Geometry: final body of the model. Coordinates: model frame, mm. A direction names the side the tool comes from. Round coordinates to 2 decimals unless told otherwise and drop trailing zeros. Write each loop counter-clockwise with the first axis right and the second up, starting at its lowest first coordinate (ties: lowest second). Pieces come first, ordered by that corner, then holes. Notation, with made-up numbers: M 10.5,35 L 66.5,35 A20 cw 66.5,57 Z; hole C 66,80.25 d9. An arc over 180 degrees is marked long. Put each result on its own line as item: value. Start each with the question number.
```python
from build123d import *

# Parameters (mm, degrees)
SKETCH_3_R          = 5
CUT_EXTRUDE_1_DEPTH = 93.736184955
CUT_EXTRUDE_2_DEPTH = 15
CUT_EXTRUDE_3_DEPTH = 15
CUT_EXTRUDE_START   = -15
CUT_EXTRUDE_4_DEPTH = 15
CUT_EXTRUDE_5_DEPTH = 15


with BuildPart() as part:
    # 扫描1: sweep along a path in 草图2
    with BuildLine(Plane.XY) as sweep_1_path:
        CenterArc((0, 0), 50, 0, 360)
    # 草图1 → 扫描1 (sweep)
    with BuildSketch(Plane(origin=(0, 0, 0), x_dir=(1, 0, 0), z_dir=(0, 1, 0))):
        with BuildLine():
            Line((0, 0), (7.5, 0))
            Line((7.5, 0), (7.5, 35))
            ThreePointArc((7.5, 35), (13.357864376, 49.142135624), (27.5, 55))
            Line((27.5, 55), (50, 55))
            Line((50, 55), (50, 60))
            Line((50, 60), (0, 60))
            Line((0, 60), (0, 0))
        make_face()
    sweep(path=sweep_1_path.line)

    # 草图3 → 切除-拉伸1 (cut, through all)
    with BuildSketch(Plane.XY):
        Circle(SKETCH_3_R)
    extrude(amount=-CUT_EXTRUDE_1_DEPTH, mode=Mode.SUBTRACT)

    # 草图5 → 切除-拉伸2 (cut)
    with BuildSketch(Plane.XY):
        Polygon((0, 7.5), (0.5, 7.5), (0, 0), align=None)
    extrude(amount=-CUT_EXTRUDE_2_DEPTH, mode=Mode.SUBTRACT)

    # 草图6 → 切除-拉伸3 (cut)
    with BuildSketch(Plane.XY):
        Polygon((0, 0), (5.303300859, 5.303300859), (5.656854249, 4.949747468), align=None)
    extrude(amount=-CUT_EXTRUDE_3_DEPTH, mode=Mode.SUBTRACT)

    # 草图8 → 切除-拉伸4 (cut)
    with BuildSketch(Plane.XY.offset(CUT_EXTRUDE_START)):
        with BuildLine():
            Line((0, 0), (0, -7.5))
            ThreePointArc((0, -7.5), (-0.249584525, -7.495846021), (-0.498892579, -7.483388684))
            Line((-0.498892579, -7.483388684), (0, 0))
        make_face()
    extrude(amount=CUT_EXTRUDE_4_DEPTH, mode=Mode.SUBTRACT)

    # 草图9 → 切除-拉伸5 (cut)
    with BuildSketch(Plane.XY.offset(CUT_EXTRUDE_START)):
        with BuildLine():
            Line((0, 0), (-5.303300859, -5.303300859))
            ThreePointArc((-5.303300859, -5.303300859), (-5.476846462, -5.123880642), (-5.64432521, -4.938784559))
            Line((-5.64432521, -4.938784559), (0, 0))
        make_face()
    extrude(amount=CUT_EXTRUDE_5_DEPTH, mode=Mode.SUBTRACT)

    # 扫描2: sweep along a curve in space
    with BuildLine() as sweep_2_path:
        ThreePointArc((5.303300859, 5.303300859, 0), (3.099122118, 6.829746854, 0), (0.498892579, 7.483388684, 0))
    # 草图10 → 扫描2 (sweep)
    with BuildSketch(Plane(origin=(0, 0, 0), x_dir=(0, 0, 1), z_dir=(-0.997785157856609, 0.06651901052377394, 0))):
        Polygon((0, 7.483388684), (-1.999931015, 7.5), (-1.999931015, 8.3), align=None)
    sweep(path=sweep_2_path.line)

    # 扫描3: sweep along a curve in space
    with BuildLine() as sweep_3_path:
        ThreePointArc((-5.303300859, -5.303300859, 0), (-3.099122118, -6.829746854, 0), (-0.498892579, -7.483388684, 0))
    # 草图11 → 扫描3 (sweep)
    with BuildSketch(Plane(origin=(0, 0, 0), x_dir=(0, 0, -1), z_dir=(0.997785157856609, -0.06651901052377394, 0))):
        Polygon((0, -7.5), (2, -7.5), (2, -8.3), align=None)
    sweep(path=sweep_3_path.line)


solid = part.part
```
1) Draft query along Z for faces 1 (the face through (-7.493, 0.33, -17.745)), 2 (the face through (-3.2, -7, -2)), 3 (the face through (-3.3, -7.18, -1.01)), 4 (the face through (47.69, 15.02, -57.54)). Return one class per face: +Z half, -Z half, draft (parallel to the pull), parting line (faces both ways), or undercut.
2) Ray query, probe 1 along Y at (x, z) = (0, -21); probe 2 along Z at (x, y) = (3, -35). Return the intervals inside material, ascending.
3) First-contact query: pin 1 (2 mm diameter, centred on y = -6, z = -10.5, fed in from -X); pin 2 (1 mm diameter, centred on x = -6.5, z = -38, fed in from -Y); pin 3 (5 mm diameter, centred on x = -21.5, y = 37.5, fed in from +Z). Flat tips, straight axial feed; report the tip coordinate or a pass-through.
4) Section B-B, the plane z = -47. Output: boundary loops of the cut face in (x, y).
5) Section A-A, the plane z = -22. Output: boundary loops of the cut face in (x, y).
6) Access query for faces 5 (the face through (3.3, 7.18, -1.03)), 6 (the face through (-1.08, -4.88, -29.58)), 7 (the face through (0, -6, -8)), 8 (the face through (3.2, 7, -2)), 9 (the face through (0, 6, -7)). Directions: +Z, -Z, +X, -X, +Y, -Y. A direction counts if a zero-diameter tool reaches every point of the face in a straight line with its end or side. Return the directions, or none.
Solved:
1. face 1: undercut
1. face 2: undercut
1. face 3: +Z half
1. face 4: draft
2. probe 1: y = -7.5 to -5, 5 to 7.5
2. probe 2: z = -60 to -55
3. pin 1: stops at x = -5.3
3. pin 2: stops at y = -4.88
3. pin 3: stops at z = -55
4. outline: C 0,0 d23; hole C 0,0 d10
5. outline: C 0,0 d15; hole C 0,0 d10
6. face 5: +Z, +X, +Y
6. face 6: +Z, -Z
6. face 7: +Z, -Y
6. face 8: +X, +Y
6. face 9: +Z, +Y
